```python
from build123d import *

# Parameters (mm, degrees)
SKETCH1_W           = 50
SKETCH1_H           = 30
BOSS_EXTRUDE1_DEPTH = 6
SKETCH3_W           = 5
SKETCH3_H           = 30
BOSS_EXTRUDE2_DEPTH = 15
SKETCH4_R           = 2.4
CUT_EXTRUDE1_DEPTH  = 5
FILLET2_R           = 3
FILLET3_R           = 5


with BuildPart() as part:
    # Sketch1 → Boss-Extrude1 (new body)
    with BuildSketch(Plane.XY):
        with Locations((-261.5, -48)):
            Rectangle(SKETCH1_W, SKETCH1_H)
    extrude(amount=BOSS_EXTRUDE1_DEPTH)

    # Sketch3 → Boss-Extrude2 (add)
    with BuildSketch(Plane.XY.offset(6)):
        with Locations((-239, -48)):
            Rectangle(SKETCH3_W, SKETCH3_H)
        with Locations((-284, -48)):
            Rectangle(SKETCH3_W, SKETCH3_H)
    extrude(amount=BOSS_EXTRUDE2_DEPTH)

    # Sketch4 → Cut-Extrude1 (cut)
    with BuildSketch(Plane(origin=(-236.5, 0, 0), x_dir=(0, 0, -1), z_dir=(1, 0, 0))):
        with Locations((-13.5, -48)):
            Circle(SKETCH4_R)
    extrude(amount=-CUT_EXTRUDE1_DEPTH, mode=Mode.SUBTRACT)

    # Fillet2
    fillet2_edges = [part.edges().sort_by_distance(p)[0] for p in [
        (-236.5, -48, 0),
        (-286.5, -48, 0),
    ]]
    fillet(fillet2_edges, radius=FILLET2_R)

    # Fillet3
    fillet3_edges = [part.edges().sort_by_distance(p)[0] for p in [
        (-239, -33, 21),
        (-239, -63, 21),
        (-284, -63, 21),
        (-284, -33, 21),
    ]]
    fillet(fillet3_edges, radius=FILLET3_R)


solid = part.part
```
Check sheet for the modelled part. Datum: model origin and axes. Units: mm. A direction names the side the tool comes from. Round coordinates to 2 decimals unless told otherwise and drop trailing zeros. Loops run counter-clockwise (first coordinate to the right, second up) from the corner with the lowest first, then second, coordinate; pieces in that order, holes last. Notation, with made-up numbers: (-14.75, 50) -> (19.25, 50) arc R17 cw to (19.25, 60) -> close; hole circle Ø11 at (54.5, -31). An arc over 180 degrees is marked (long way). Answer in a Markdown table with one row per item.
Q1. Sectioned sample at C-C on x = -241. Enter the section's corners in (y, z).
Data:
| item | result |
|---|---|
| outline | (-63, 0) -> (-33, 0) -> (-33, 16) arc R5 ccw to (-38, 21) -> (-58, 21) arc R5 ccw to (-63, 16) -> close; hole circle Ø4.8 at (-48, 13.5) |
Q2. Sectioned sample at B-B on z = 13.5. Enter the section's corners in (x, y), then the cut area to 3 significant figures.
Data:
| item | result |
|---|---|
| outline | (-286.5, -63) -> (-281.5, -63) -> (-281.5, -33) -> (-286.5, -33) -> close; (-241.5, -63) -> (-236.5, -63) -> (-236.5, -50.4) -> (-241.5, -50.4) -> close; (-241.5, -45.6) -> (-236.5, -45.6) -> (-236.5, -33) -> (-241.5, -33) -> close |
| area | 276 mm^2 |
Q3. Thickness scan on L1, parallel to X at y = -60.5, z = 13.5; L2, parallel to Y at x = -240.05, z = 13.5; L3, parallel to Z at x = -244, y = -51.5. Record the ranges inside material, lowest first.
Data:
| item | result |
|---|---|
| L1 | x = -286.5 to -281.5, -241.5 to -236.5 |
| L2 | y = -63 to -50.4, -45.6 to -33 |
| L3 | z = 0 to 6 |
Q4. Set-up check for faces 4 (the face through (-284, -48, 21)), 5 (the face through (-238.965, -50.343, 14.02)), 6 (the face through (-262, -48, 6)): record each of +Z, -Z, +X, -X, +Y, -Y from which the full face is reachable in a straight line by a thin tool's end or side.
Data:
| item | result |
|---|---|
| face 4 | +Z, +X, -X, +Y, -Y |
| face 5 | +X |
| face 6 | +Z, +Y, -Y |
Q5. Sectioned sample at A-A on y = -48. Enter the section's corners in (x, z).
Data:
| item | result |
|---|---|
| outline | (-286.5, 3) arc R3 ccw to (-283.5, 0) -> (-239.5, 0) arc R3 ccw to (-236.5, 3) -> (-236.5, 11.1) -> (-241.5, 11.1) -> (-241.5, 6) -> (-281.5, 6) -> (-281.5, 21) -> (-286.5, 21) -> close; (-241.5, 15.9) -> (-236.5, 15.9) -> (-236.5, 21) -> (-241.5, 21) -> close |
Q6. Go/stop test with a flat-tipped pin: P1, Ø1, axis at x = -272.5, y = -54.5, coming from the +Z side. Record where the tip stops, or that it passes through.
Data:
| item | result |
|---|---|
| P1 | stops at z = 6 |
Q7. Release check for a two-part mould opening along X. For faces 1 (the face through (-286.5, -48, 12)), 2 (the face through (-239, -62, 19)), 3 (the face through (-241.5, -48, 10)) record: released by +X, released by -X, zero draft, split by the parting line, or undercut.
Data:
| item | result |
|---|---|
| face 1 | released by -X |
| face 2 | zero draft |
| face 3 | undercut |
Q8. Sectioned sample at D-D on z = 16.5. Enter the section's corners in (x, y).
Data:
| item | result |
|---|---|
| outline | (-286.5, -62.97) -> (-281.5, -62.97) -> (-281.5, -33.03) -> (-286.5, -33.03) -> close; (-241.5, -62.97) -> (-236.5, -62.97) -> (-236.5, -33.03) -> (-241.5, -33.03) -> close |
